from build123d import *

# Parameters (mm, degrees)
SKETCH_2_OUTSIDE_W  = 16.808
SKETCH_2_OUTSIDE_H  = 16.808
CUT_EXTRUDE_1_DEPTH = 12


with BuildPart() as part:
    # Эскиз1 → Повернуть1 (revolve)
    with BuildSketch(Plane.XY):
        Polygon((-4, 0), (-4, 4.75), (-3.812435565, 5.45), (0, 5.45), (0, 3), (7.4, 3), (8, 2.4), (8, 0), align=None)
    revolve(axis=Axis((-1000, 0, 0), (1, 0, 0)))

    # Эскиз2 outside → Вырез-Вытянуть1 (cut)
    with BuildSketch(Plane.ZY.offset(4)):
        Rectangle(SKETCH_2_OUTSIDE_W, SKETCH_2_OUTSIDE_H)
        Polygon((0, 5.773502692), (-5, 2.886751346), (-5, -2.886751346), (0, -5.773502692), (5, -2.886751346), (5, 2.886751346), align=None, mode=Mode.SUBTRACT)
    extrude(amount=-CUT_EXTRUDE_1_DEPTH, mode=Mode.SUBTRACT)


solid = part.part
Check sheet for the modelled part. Datum: model origin and axes. Units: mm. A direction names the side the tool comes from. Round coordinates to 2 decimals unless told otherwise and drop trailing zeros. Loops run counter-clockwise (first coordinate to the right, second up) from the corner with the lowest first, then second, coordinate; pieces in that order, holes last. Notation, with made-up numbers: M -16.75,74.25 L 16.25,74.25 A19 cw 16.25,89.25 Z; hole C 50.25,7.25 d1. An arc over 180 degrees is marked long. One line per item, written item: value.
(1) Sectioned sample at B-B, the plane x = -1.25. Record the cut outline in (y, z), then the cut area to 3 significant figures.
Computed values:
outline: M -5.41,-0.62 L -3.25,-4.38 A5.45 ccw -2.17,-5 L 2.17,-5 A5.45 ccw 3.25,-4.38 L 5.41,-0.62 A5.45 ccw 5.41,0.62 L 3.25,4.38 A5.45 ccw 2.17,5 L -2.17,5 A5.45 ccw -3.25,4.38 L -5.41,0.62 A5.45 ccw Z
area: 85.4 mm^2
(2) Access from +Z, -Z, +X, -X, +Y, -Y to the whole of each face (thin tool, end or side, straight path). Record for faces 1 (the face through (4, -3, 0)), 2 (the face through (-2, 0, 5)).
Computed values:
face 1: +X
face 2: +Z, +X, -X, +Y, -Y
(3) Sectioned sample at C-C, the plane x = 1.5. Record the cut outline in (y, z).
Computed values:
outline: C 0,0 d6
(4) Thickness scan on line 1 (X direction, y = -4, z = 2.5); line 2 (Z direction, x = -1.25, y = -4.5); line 3 (Y direction, x = 2.25, z = -1.25). Record the ranges inside material, lowest first.
Computed values:
line 1: x = -4 to 0
line 2: z = -2.21 to 2.21
line 3: y = -2.73 to 2.73
(5) Depth check by flat-ended pin: pin 1 Ø1.5 at (x, y) = (2.5, -2.5) entering from +Z; pin 2 Ø2 at (x, z) = (-0.5, 3.5) entering from -Y; pin 3 Ø1.5 at (x, z) = (-0.5, -3) entering from +Y. Enter the tip coordinate at first touch or a pass-through.
Computed values:
pin 1: stops at z = 2.44
pin 2: stops at y = -4.33
pin 3: stops at y = 4.47
(6) Sectioned sample at A-A, the plane z = 0. Record the cut outline in (x, y), then the cut area to 3 significant figures.
Computed values:
outline: M -4,-4.75 L -3.81,-5.45 L 0,-5.45 L 0,-3 L 7.4,-3 L 8,-2.4 L 8,2.4 L 7.4,3 L 0,3 L 0,5.45 L -3.81,5.45 L -4,4.75 Z
area: 91.1 mm^2
